Check sheet for the drawn part. Datum: minimum x, y, z corner. Units: mm. Round coordinates to 2 decimals unless told otherwise and drop trailing zeros. Loops run counter-clockwise (first coordinate to the right, second up) from the corner with the lowest first, then second, coordinate; pieces in that order, holes last.
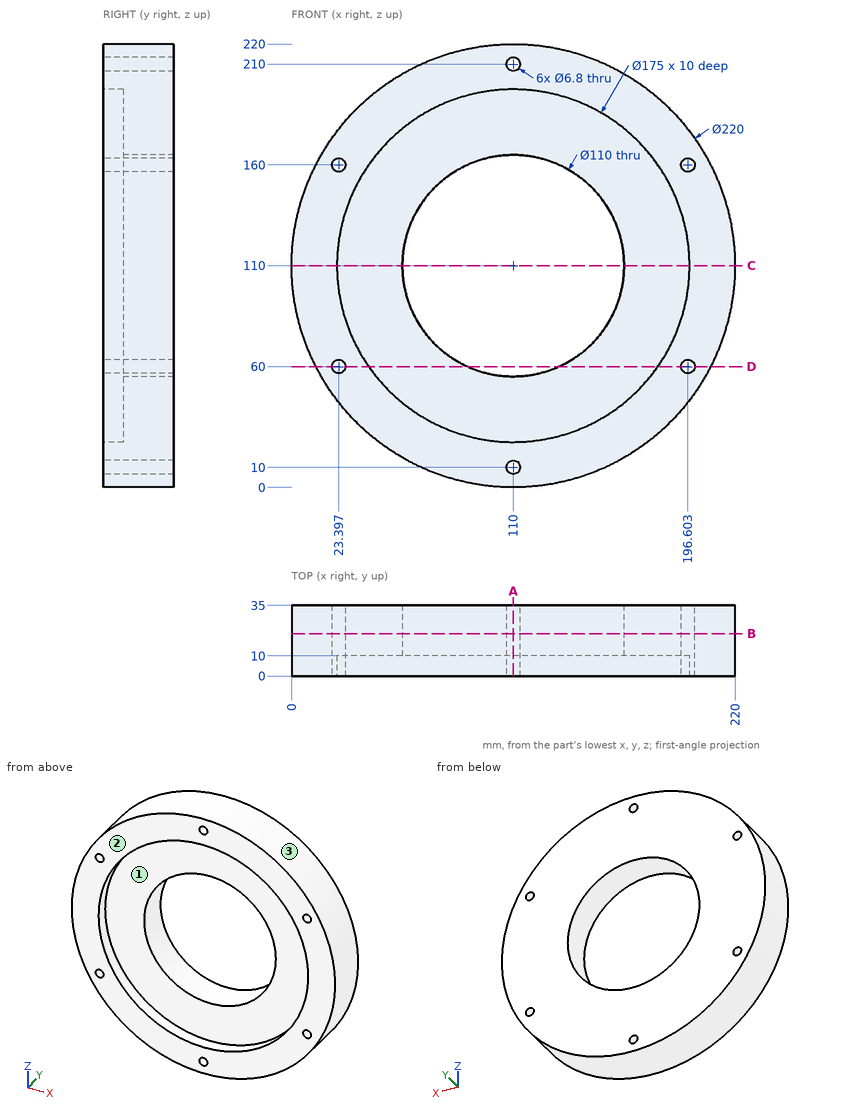
1. Section check A-A (x = 110). Enter the section's corners in (y, z).
2. Section check B-B (y = 21). Enter the section's corners in (x, z).
3. Section check C-C (z = 110). Enter the section's corners in (x, y).
4. Section check D-D (z = 60). Enter the section's corners in (x, y), then the cut area to 3 significant figures.
5. Gauge pin test, flat ends, axial feed: P1, Ø4, axis at x = 97, y = 22.5, coming from the +Z side; P2, Ø12, axis at y = 25.5, z = 66, coming from the +X side; P3, Ø10, axis at x = 130, y = 5, coming from the +Z side. Record the tip position at first contact, or that the pin passes through.
6. Scan lines: L1, parallel to Z at x = 110, y = 11.5; L2, parallel to X at y = 27, z = 60 (1 decimal); L3, parallel to X at y = 17, z = 110. Record each from-to range of solid material in increasing order.
7. Release check for a two-part mould opening along X. For the marked faces 1, 2 and 3 record: released by +X, released by -X, zero draft, split by the parting line, or undercut.
Taken from the geometry:
1. outline: (0, 0) - (35, 0) - (35, 6.6) - (0, 6.6) - close; (0, 13.4) - (35, 13.4) - (35, 55) - (10, 55) - (10, 22.5) - (0, 22.5) - close; (0, 197.5) - (10, 197.5) - (10, 165) - (35, 165) - (35, 206.6) - (0, 206.6) - close; (0, 213.4) - (35, 213.4) - (35, 220) - (0, 220) - close
2. outline: circle Ø220 at (110, 110); hole circle Ø6.8 at (23.4, 60); hole circle Ø6.8 at (23.4, 160); hole circle Ø110 at (110, 110); hole circle Ø6.8 at (110, 10); hole circle Ø6.8 at (110, 210); hole circle Ø6.8 at (196.6, 60); hole circle Ø6.8 at (196.6, 160)
3. outline: (0, 0) - (22.5, 0) - (22.5, 10) - (55, 10) - (55, 35) - (0, 35) - close; (165, 10) - (197.5, 10) - (197.5, 0) - (220, 0) - (220, 35) - (165, 35) - close
4. outline: (12.02, 0) - (20, 0) - (20, 35) - (12.02, 35) - close; (26.8, 0) - (38.19, 0) - (38.19, 10) - (87.09, 10) - (87.09, 35) - (26.8, 35) - close; (132.91, 10) - (181.81, 10) - (181.81, 0) - (193.2, 0) - (193.2, 35) - (132.91, 35) - close; (200, 0) - (207.98, 0) - (207.98, 35) - (200, 35) - close
4. area: 3,800 mm2
5. P1: stops at z = 219.45
5. P2: stops at x = 213.23
5. P3: stops at z = 218.97
6. L1: z = 0 to 6.6, 13.4 to 55, 165 to 206.6, 213.4 to 220
6. L2: x = 12 to 20, 26.8 to 87.1, 132.9 to 193.2, 200 to 208
6. L3: x = 0 to 55, 165 to 220
7. face 1: undercut
7. face 2: zero draft
7. face 3: split by the parting line
